Geometry: final body of the model. Coordinates: model frame, mm. A direction names the side the tool comes from. Round coordinates to 2 decimals unless told otherwise and drop trailing zeros. Loops run counter-clockwise (first coordinate to the right, second up) from the corner with the lowest first, then second, coordinate; pieces in that order, holes last. Notation, with made-up numbers: (31, 84.25) -> (51, 84.25) arc R24 ccw to (51, 109.25) -> close; hole circle Ø11 at (-21, 71.25). An arc over 180 degrees is marked (long way). Answer in a Markdown table with one row per item.
Autodesk Inventor part; units mm, degrees
ref_plane "YZ Plane" through (0, 0, 0) normal (1, 0, 0) x (0, 1, 0)
ref_plane "XZ Plane" through (0, 0, 0) normal (0, 1, 0) x (-1, 0, 0)
ref_plane "XY Plane" through (0, 0, 0) normal (0, 0, 1) x (1, 0, 0)
sketch "草图1" plane through (0, 0, 0) normal (0, 0, 1) x (1, 0, 0)
  line L0 (0, 0) -> (40, 0)
  line L1 (40, 0) -> (40, -26)
  line L2 (40, -26) -> (0, -26)
  line L3 (0, -26) -> (0, 0)
  dimension "d0" = 40
  dimension "d1" = 26
extrude "拉伸1" add sketch "草图1" along normal blind 10
ref_plane "工作平面1" through (20, -26, 0) normal (1, 0, 0) x (0, 0, -1)
sketch "草图2" plane through (20, -26, 0) normal (1, 0, 0) x (0, 0, -1)
  line L0 (0, 26) -> (-10, 26)
  line L1 (0, 26) -> (-10, 26)
  line L2 (-10, 26) -> (-10, 38)
  line L3 (-10, 38) -> (0, 38)
  line L4 (0, 38) -> (0, 26)
  line L5 (-10, 38) -> (-41, 38)
  line L6 (-41, 38) -> (-41, 34.5)
  line L7 (-41, 34.5) -> (-10, 34.5)
  line L8 (-10, 34.5) -> (-10, 38)
  line L9 (-41, 34.5) -> (-31, 34.5)
  line L10 (-31, 34.5) -> (-31, 30.5)
  line L11 (-31, 30.5) -> (-41, 30.5)
  line L12 (-41, 30.5) -> (-41, 34.5)
  dimension "d5" = 10
  dimension "d6" = 12
  dimension "d7" = 31
  dimension "d8" = 3.5
  dimension "d9" = 10
  dimension "d10" = 4
extrude "拉伸2" add sketch "草图2" along normal mid plane 20
sketch "草图3" plane through (0, 0, 0) normal (0, 0, -1) x (-1, 0, 0)
  line L0 (-30, -11) -> (-10, -11)
  line L1 (-10, -11) -> (-10, -15)
  line L2 (-10, -15) -> (-30, -15)
  line L3 (-30, -15) -> (-30, -11)
  line L4 (-40, 0) -> (-30, 0)
  line L5 (-40, -26) -> (-40, 0)
  line L6 (-30, -11) -> (-10, -11)
  line L7 (-10, -11) -> (-10, -6)
  line L8 (-10, -6) -> (-30, -6)
  line L9 (-30, -6) -> (-30, -11)
  line L10 (-30, -15) -> (-10, -15)
  line L11 (-10, -15) -> (-10, -20)
  line L12 (-10, -20) -> (-30, -20)
  line L13 (-30, -20) -> (-30, -15)
  point P0 (0, 0)
  dimension "d13" = 20
  dimension "d14" = 4
  dimension "d15" = 11
  dimension "d16" = 10
  dimension "d17" = 5
  dimension "d18" = 20
  dimension "d19" = 5
extrude "拉伸3" add sketch "草图3" along normal blind 13 contours L9 L8 L7 L0 | L2 L11 L12 L13
fillet "圆角1" radius 5 6 edges at (30, -8.5, 0) (20, -6, 0) (10, -8.5, 0) (10, -17.5, 0) (20, -20, 0) (30, -17.5, 0)
fillet "圆角2" radius 5 2 edges at (20, 12, 0) (20, 8.5, 10)
properties part number "连接件"
Item 1: Cut plane D-D (z = 1). Output: boundary loops of the cut face in (x, y).
Answer:
| item | result |
|---|---|
| outline | (0, -26) -> (40, -26) -> (40, 0) -> (30, 0) -> (30, 10) -> (10, 10) -> (10, 0) -> (0, 0) -> close |
Item 2: Line query: probe 1 along X at (y, z) = (6.5, 35); probe 2 along Y at (x, z) = (14, 15); probe 3 along Z at (x, y) = (3, -1). Output: solid intervals per line, ascending. Write a range as [from, to].
Answer:
| item | result |
|---|---|
| probe 1 | x = [10, 30] |
| probe 2 | y = [8.5, 12] |
| probe 3 | z = [0, 10] |
Item 3: Reachability of faces 5 (the face through (20, 7, 31)), 6 (the face through (20, -6, -9)), 7 (the face through (30, 9, 21)) from +Z, -Z, +X, -X, +Y, -Y: full face, straight path, thin tool, end or side. Return the list, or none.
Answer:
| item | result |
|---|---|
| face 5 | +X, -X, -Y |
| face 6 | -Z, +X, -X, +Y |
| face 7 | +Z, -Z, +X, +Y |
Item 4: Cut plane B-B (x = 27.5). Output: boundary loops of the cut face in (y, z).
Answer:
| item | result |
|---|---|
| outline | (-26, 0) -> (-25, 0) arc R5 cw to (-20, -5) -> (-20, -13) -> (-15, -13) -> (-15, 0) -> (-11, 0) -> (-11, -13) -> (-6, -13) -> (-6, -5) arc R5 cw to (-1, 0) -> (7, 0) arc R5 ccw to (12, 5) -> (12, 41) -> (4.5, 41) -> (4.5, 31) -> (8.5, 31) -> (8.5, 15) arc R5 cw to (3.5, 10) -> (-26, 10) -> close |
Item 5: Cut plane C-C (y = -10). Output: boundary loops of the cut face in (x, z).
Answer:
| item | result |
|---|---|
| outline | (0, 0) -> (5, 0) arc R5 cw to (10, -5) -> (10, -13) -> (30, -13) -> (30, -5) arc R5 cw to (35, 0) -> (40, 0) -> (40, 10) -> (0, 10) -> close |
Item 6: Draft query along Z for faces 1 (the face through (19.86, 7.07, 11.5)), 2 (the face through (20, 12, 23)), 3 (the face through (20, 8, 41)), 4 (the face through (20, 8.5, 23)). Return one class per face: pulls with the +Z half, pulls with the -Z half, needs draft (parallel to the pull), parting line crosses it, or undercut.
Answer:
| item | result |
|---|---|
| face 1 | undercut |
| face 2 | needs draft |
| face 3 | pulls with the +Z half |
| face 4 | undercut |
Item 7: Cut plane A-A (z = -7). Output: boundary loops of the cut face in (x, y).
Answer:
| item | result |
|---|---|
| outline | (10, -20) -> (30, -20) -> (30, -15) -> (10, -15) -> close; (10, -11) -> (30, -11) -> (30, -6) -> (10, -6) -> close |
Item 8: Pin query (flat end, axial travel): pin 1 Ø4 at (x, z) = (24, -9.5) entering from +Y; pin 2 Ø1.5 at (y, z) = (-17.5, -9.5) entering from +X; pin 3 Ø17.5 at (x, z) = (23, 24.5) entering from -Y. Return the tip coordinate at first contact, or that it passes through.
Answer:
| item | result |
|---|---|
| pin 1 | stops at y = -6 |
| pin 2 | stops at x = 30 |
| pin 3 | stops at y = 4.5 |
